```python
from build123d import *

# Parameters (mm, degrees)
CHAMFER_1_SIZE = 1
CHAMFER_2_SIZE = 3
CHAMFER_3_SIZE = 1


with BuildPart() as part:
    # Эскиз1 → Повернуть1 (revolve)
    with BuildSketch(Plane.XY, mode=Mode.PRIVATE) as revolve_1_sk:
        Polygon((0, 20), (0, 74.59), (4, 74.59), (4, 69.89), (11.3, 69.89), (11.3, 74.59), (15.3, 74.59), (15.3, 73.09), (25, 73.09), (25, 74.59), (29, 74.59), (29, 69.89), (36.3, 69.89), (36.3, 74.59), (40.3, 74.59), (40.3, 20), (37.3, 20), (37.3, 9), (15, 9), (15, 20), align=None)
    revolve(revolve_1_sk.sketch.rotate(Axis((0, 0, 0), (-1, 0, 0)), 90), axis=Axis((0, 0, 0), (-1, 0, 0)))

    # Фаска1
    chamfer_1_edges = [part.edges().sort_by_distance(p)[0] for p in [
        (40.3, 0, 74.59),
        (0, 0, 74.59),
    ]]
    chamfer(chamfer_1_edges, length=CHAMFER_1_SIZE)

    # Фаска2
    chamfer_2_edges = [part.edges().sort_by_distance(p)[0] for p in [
        (15, 0, 20),
    ]]
    chamfer(chamfer_2_edges, length=CHAMFER_2_SIZE)

    # Фаска3
    chamfer_3_edges = [part.edges().sort_by_distance(p)[0] for p in [
        (37.3, 0, 20),
        (0, 0, 20),
    ]]
    chamfer(chamfer_3_edges, length=CHAMFER_3_SIZE)


solid = part.part
```
Can you work these out from the model? Positions are in its coordinate system, mm. A direction names the side the tool comes from. Coordinates: 2 decimals unless noted, no trailing zeros. Loops run counter-clockwise (first coordinate to the right, second up) from the corner with the lowest first, then second, coordinate; pieces in that order, holes last.
1) I need wall thicknesses on probe 1 along Y at (x, z) = (20, 0); probe 2 along Y at (x, z) = (5.5, 0); probe 3 along Z at (x, y) = (28, 3.5). Which ranges of each line are inside material? Lowest first, please.
2) Thinking about a two-plate mould opening in X: for faces 5 (the cylindrical face through (32.7, 68.23, 15.15)), 6 (the flat face through (40.3, 15, -15)), 7 (the cylindrical face through (27.028, 72.816, 16.17)), 8 (the cylindrical face through (20.2, -22, -69.7)), which applies, pulls with the +X half, pulls with the -X half, needs draft (parallel to the pull), parting line crosses it, or undercut?
3) Which directions (+Z, -Z, +X, -X, +Y, -Y) give clear straight access to the entire face, cutting with the end or side of a thin tool? Please do faces 1 (the flat face through (37.3, -4.5, -8.2)), 2 (the cylindrical face through (2.521, 72.816, 16.17)), 3 (the cylindrical face through (6.42, -0.88, 19.98)), 4 (the flat face through (15.3, 49, -55)).
4) For pin 1 (5 mm diameter, centred on x = 15, z = -48, fed in from +Y); pin 2 (17 mm diameter, centred on y = -6.5, z = -3, fed in from -X); pin 3 (4 mm diameter, centred on x = 12.5, z = -43, fed in from +Y), each with a flat end and sliding along its axis, tell me the tip position at first contact or that it passes through.
5) Imagine slicing it at A-A on x = 9. List the corners of the cut face in (y, z) for me, plus the area to 3 significant figures.
6) Imagine slicing it at B-B on x = 21. List the corners of the cut face in (y, z) for me.
Completed:
1. probe 1: y = -73.09 to -9, 9 to 73.09
1. probe 2: y = -69.89 to -20, 20 to 69.89
1. probe 3: z = -74.51 to -8.29, 8.29 to 74.51
2. face 5: undercut
2. face 6: pulls with the +X half
2. face 7: needs draft
2. face 8: undercut
3. face 1: +X
3. face 2: +X, -X
3. face 3: -X
3. face 4: none
4. pin 1: stops at y = 59.11
4. pin 2: stops at x = 15
4. pin 3: stops at y = 62.31
5. outline: circle Ø139.78 at (0, 0); hole circle Ø40 at (0, 0)
5. area: 14,100 mm2
6. outline: circle Ø146.18 at (0, 0); hole circle Ø18 at (0, 0)
